```python
from build123d import *

# Parameters (mm, degrees)
SKETCH1_W           = 6.35
SKETCH1_H           = 203.2
SKETCH1_W_2         = 4.7625
SKETCH1_H_2         = 29.028571429
BOSS_EXTRUDE1_DEPTH = 4.7625
SKETCH2_W           = 4.7625
SKETCH2_H           = 203.2
BOSS_EXTRUDE2_DEPTH = 13.5


with BuildPart() as part:
    # Sketch1 → Boss-Extrude1 (new body)
    with BuildSketch(Plane.XY):
        with Locations((-3.175, 0)):
            Rectangle(SKETCH1_W, SKETCH1_H)
        Polygon((6.35, 101.6), (0, 101.6), (0, -101.6), (6.35, -101.6), (6.35, -72.571428571), (6.35, -43.542857143), (6.35, -14.514285714), (6.35, 14.514285714), (6.35, 43.542857143), (6.35, 72.571428571), align=None)
        with Locations((8.73125, 87.085714286)):
            Rectangle(SKETCH1_W_2, SKETCH1_H_2)
        with Locations((8.73125, 29.028571429)):
            Rectangle(SKETCH1_W_2, SKETCH1_H_2)
        with Locations((8.73125, -29.028571429)):
            Rectangle(SKETCH1_W_2, SKETCH1_H_2)
        with Locations((8.73125, -87.085714286)):
            Rectangle(SKETCH1_W_2, SKETCH1_H_2)
    extrude(amount=BOSS_EXTRUDE1_DEPTH)

    # Sketch2 → Boss-Extrude2 (add)
    with BuildSketch(Plane.ZY.offset(6.35)):
        with Locations((2.38125, 0)):
            Rectangle(SKETCH2_W, SKETCH2_H)
    extrude(amount=BOSS_EXTRUDE2_DEPTH)


solid = part.part
```
Work out the finished part from the listing and answer in its coordinate system (mm). A direction names the side the tool comes from. Coordinates: 2 decimals unless noted, no trailing zeros. Write each loop counter-clockwise with the first axis right and the second up, starting at its lowest first coordinate (ties: lowest second). Pieces come first, ordered by that corner, then holes.
Q1. Determine the mould class of faces 1 (the face through (-4, -1, 4.762)), 2 (the face through (-4, -101.6, 2)), 3 (the face through (-4, 101.6, 2)), 4 (the face through (9, -72.571, 2)) for opening direction Y: released by +Y, released by -Y, zero draft, split by the parting line, or undercut.
Q2. A cutting plane is placed at A-A, the plane x = 8. Give the vertices of the cut face in (y, z).
Q3. Find the intervals of material crossed by line 1 (Y direction, x = 9, z = 4); line 2 (X direction, y = -2, z = 2.5), in increasing order.
Q4. Which of the six approach directions +Z, -Z, +X, -X, +Y, -Y give full straight-line access (tool end or side, diameter ignored) to faces 5 (the face through (9, -43.543, 2)), 6 (the face through (-19.85, 1, 2))?
Q5. A cutting plane is placed at B-B, the plane z = 1.35. Give the vertices of the cut face in (x, y), then the cut area to 3 significant figures.
Q6. Each of these flat-tipped pins is pushed along its axis until it touches: pin 1 Ø1.4 at (y, z) = (-62, 1.5) entering from +X; pin 2 Ø1 at (y, z) = (-44, 1) entering from +X. Where does it stop, or does it pass through?
Q7. A cutting plane is placed at C-C, the plane y = 53. Give the vertices of the cut face in (x, z).
Findings below:
1. face 1: zero draft
1. face 2: released by -Y
1. face 3: released by +Y
1. face 4: undercut
2. outline: (-101.6, 0) - (-72.57, 0) - (-72.57, 4.76) - (-101.6, 4.76) - close; (-43.54, 0) - (-14.51, 0) - (-14.51, 4.76) - (-43.54, 4.76) - close; (14.51, 0) - (43.54, 0) - (43.54, 4.76) - (14.51, 4.76) - close; (72.57, 0) - (101.6, 0) - (101.6, 4.76) - (72.57, 4.76) - close
3. line 1: y = -101.6 to -72.57, -43.54 to -14.51, 14.51 to 43.54, 72.57 to 101.6
3. line 2: x = -19.85 to 6.35
4. face 5: +Z, -Z, +X
4. face 6: +Z, -Z, -X, +Y, -Y
5. outline: (-19.85, -101.6) - (11.11, -101.6) - (11.11, -72.57) - (6.35, -72.57) - (6.35, -43.54) - (11.11, -43.54) - (11.11, -14.51) - (6.35, -14.51) - (6.35, 14.51) - (11.11, 14.51) - (11.11, 43.54) - (6.35, 43.54) - (6.35, 72.57) - (11.11, 72.57) - (11.11, 101.6) - (-19.85, 101.6) - close
5. area: 5,880 mm2
6. pin 1: stops at x = 6.35
6. pin 2: stops at x = 11.11
7. outline: (-19.85, 0) - (6.35, 0) - (6.35, 4.76) - (-19.85, 4.76) - close
